```python
from build123d import *

# Parameters (mm, degrees)
SKETCH1_W           = 86.35
SKETCH1_H           = 86
SKETCH1_R           = 2.05
BOSS_EXTRUDE1_DEPTH = 3.175
FILLET1_R           = 4
SKETCH2_R           = 7.05
SKETCH2_R_2         = 12
CUT_EXTRUDE1_DEPTH  = 3.18


with BuildPart() as part:
    # Sketch1 → Boss-Extrude1 (new body)
    with BuildSketch(Plane(origin=(0, 0, 0), x_dir=(1, 0, 0), z_dir=(0, 1, 0))):
        Rectangle(SKETCH1_W, SKETCH1_H)
        with Locations(Location((37.675, 35, 0), (0, 0, 270))):
            Circle(SKETCH1_R, mode=Mode.SUBTRACT)
        with Locations(Location((37.675, 26.832661921, 0), (0, 0, 270))):
            Circle(SKETCH1_R, mode=Mode.SUBTRACT)
        with Locations(Location((37.675, 18.665323842, 0), (0, 0, 270))):
            Circle(SKETCH1_R, mode=Mode.SUBTRACT)
        with Locations(Location((37.675, 10.497985763, 0), (0, 0, 270))):
            Circle(SKETCH1_R, mode=Mode.SUBTRACT)
        with Locations(Location((37.675, 2.330647684, 0), (0, 0, 270))):
            Circle(SKETCH1_R, mode=Mode.SUBTRACT)
        with Locations(Location((37.675, -5.836690395, 0), (0, 0, 270))):
            Circle(SKETCH1_R, mode=Mode.SUBTRACT)
        with Locations(Location((37.675, -14.004028475, 0), (0, 0, 270))):
            Circle(SKETCH1_R, mode=Mode.SUBTRACT)
        with Locations(Location((37.675, -22.171366554, 0), (0, 0, 270))):
            Circle(SKETCH1_R, mode=Mode.SUBTRACT)
        with Locations(Location((37.675, -30.338704633, 0), (0, 0, 270))):
            Circle(SKETCH1_R, mode=Mode.SUBTRACT)
        with Locations(Location((37.675, -38.506042712, 0), (0, 0, 270))):
            Circle(SKETCH1_R, mode=Mode.SUBTRACT)
        with Locations(Location((-37.675, -38.506042712, 0), (0, 0, 90))):
            Circle(SKETCH1_R, mode=Mode.SUBTRACT)
        with Locations(Location((-37.675, -30.338704633, 0), (0, 0, 90))):
            Circle(SKETCH1_R, mode=Mode.SUBTRACT)
        with Locations(Location((-37.675, -22.171366554, 0), (0, 0, 90))):
            Circle(SKETCH1_R, mode=Mode.SUBTRACT)
        with Locations(Location((-37.675, -14.004028475, 0), (0, 0, 90))):
            Circle(SKETCH1_R, mode=Mode.SUBTRACT)
        with Locations(Location((-37.675, -5.836690395, 0), (0, 0, 90))):
            Circle(SKETCH1_R, mode=Mode.SUBTRACT)
        with Locations(Location((-37.675, 2.330647684, 0), (0, 0, 90))):
            Circle(SKETCH1_R, mode=Mode.SUBTRACT)
        with Locations(Location((-37.675, 10.497985763, 0), (0, 0, 90))):
            Circle(SKETCH1_R, mode=Mode.SUBTRACT)
        with Locations(Location((-37.675, 18.665323842, 0), (0, 0, 90))):
            Circle(SKETCH1_R, mode=Mode.SUBTRACT)
        with Locations(Location((-37.675, 26.832661921, 0), (0, 0, 90))):
            Circle(SKETCH1_R, mode=Mode.SUBTRACT)
        with Locations(Location((-37.675, 35, 0), (0, 0, 90))):
            Circle(SKETCH1_R, mode=Mode.SUBTRACT)
    extrude(amount=BOSS_EXTRUDE1_DEPTH)

    # Fillet1
    fillet1_edges = [part.edges().sort_by_distance(p)[0] for p in [
        (43.175, 1.5875, 43),
        (-43.175, 1.5875, 43),
        (-43.175, 1.5875, -43),
        (43.175, 1.5875, -43),
    ]]
    fillet(fillet1_edges, radius=FILLET1_R)

    # Sketch2 → Cut-Extrude1 (cut)
    with BuildSketch(Plane(origin=(0, 3.175, 0), x_dir=(1, 0, 0), z_dir=(0, 1, 0))):
        with Locations(Location((-17.9, 23, 0), (0, 0, 270))):
            Circle(SKETCH2_R)
        with Locations(Location((17.9, 23, 0), (0, 0, 270))):
            Circle(SKETCH2_R)
        with Locations(Location((0, -20.993410297, 0), (0, 0, 270))):
            Circle(SKETCH2_R_2)
        with BuildLine():
            Line((-17.9, -7.043410297), (-14.9, -7.043410297))
            ThreePointArc((-14.9, -7.043410297), (-12.85, -4.993410297), (-14.9, -2.943410297))
            Line((-14.9, -2.943410297), (-17.9, -2.943410297))
            ThreePointArc((-17.9, -2.943410297), (-19.95, -4.993410297), (-17.9, -7.043410297))
        make_face()
        with BuildLine():
            Line((17.1, -2.943410297), (14.1, -2.943410297))
            ThreePointArc((14.1, -2.943410297), (12.05, -4.993410297), (14.1, -7.043410297))
            Line((14.1, -7.043410297), (17.1, -7.043410297))
            ThreePointArc((17.1, -7.043410297), (19.15, -4.993410297), (17.1, -2.943410297))
        make_face()
        with BuildLine():
            Line((14.1, -34.943410297), (17.1, -34.943410297))
            ThreePointArc((17.1, -34.943410297), (19.15, -36.993410297), (17.1, -39.043410297))
            Line((17.1, -39.043410297), (14.1, -39.043410297))
            ThreePointArc((14.1, -39.043410297), (12.05, -36.993410297), (14.1, -34.943410297))
        make_face()
        with BuildLine():
            Line((-17.9, -34.943410297), (-14.9, -34.943410297))
            ThreePointArc((-14.9, -34.943410297), (-12.85, -36.993410297), (-14.9, -39.043410297))
            Line((-14.9, -39.043410297), (-17.9, -39.043410297))
            ThreePointArc((-17.9, -39.043410297), (-19.95, -36.993410297), (-17.9, -34.943410297))
        make_face()
    extrude(amount=-CUT_EXTRUDE1_DEPTH, mode=Mode.SUBTRACT)


solid = part.part
```
Source: CAD feature listing. Evaluate the final solid. Frame: model axes, mm. A direction names the side the tool comes from. Give positions to 0.01 mm unless a question says otherwise; leave off trailing zeros. Write each loop counter-clockwise with the first axis right and the second up, starting at its lowest first coordinate (ties: lowest second). Pieces come first, ordered by that corner, then holes.
1. Section query D-D (z = -1.5). Return the cut outline in (x, y) (3 decimals), then the cut area to 3 significant figures.
2. Section query B-B (z = -35). Return the cut outline in (x, y) (3 decimals), then the cut area to 3 significant figures.
3. Material intervals for line 1 along X through (y, z) = (1.2, -35) (3 decimals); line 2 along Z through (x, y) = (0.5, 1.2); line 3 along X through (y, z) = (3, 13.5) (3 decimals), sorted ascending.
4. Pull-direction query (X, two-part tool) for faces 1 (the face through (-1, 2, -43)), 2 (the face through (-43.175, 2, 1)), 3 (the face through (35.856, 1.565, 23.117)); classes: +X half, -X half, draft (parallel to the pull), parting line (faces both ways), or undercut.
5. Section query A-A (x = 0). Return the cut outline in (y, z) (3 decimals), then the cut area to 3 significant figures.
6. Section query C-C (z = 26). Return the cut outline in (x, y) (3 decimals), then the cut area to 3 significant figures.
7. Access query for faces 4 (the face through (-12.85, 1.61, 36.95)), 5 (the face through (41.97, 1.61, 41.86)). Directions: +Z, -Z, +X, -X, +Y, -Y. A direction counts if a zero-diameter tool reaches every point of the face in a straight line with its end or side. Return the directions, or none.
Output values:
1. outline: (-43.175, 0) - (-39.549, 0) - (-39.549, 3.175) - (-43.175, 3.175) - close; (-35.801, 0) - (35.801, 0) - (35.801, 3.175) - (-35.801, 3.175) - close; (39.549, 0) - (43.175, 0) - (43.175, 3.175) - (39.549, 3.175) - close
1. area: 250 mm2
2. outline: (-43.175, 0) - (-39.725, 0) - (-39.725, 3.175) - (-43.175, 3.175) - close; (-35.625, 0) - (35.625, 0) - (35.625, 3.175) - (-35.625, 3.175) - close; (39.725, 0) - (43.175, 0) - (43.175, 3.175) - (39.725, 3.175) - close
2. area: 248 mm2
3. line 1: x = -43.175 to -39.725, -35.625 to 35.625, 39.725 to 43.175
3. line 2: z = -43 to 9, 32.98 to 43
3. line 3: x = -43.175 to -39.662, -35.688 to -9.373, 9.373 to 35.688, 39.662 to 43.175
4. face 1: draft
4. face 2: -X half
4. face 3: undercut
5. outline: (0, -43) - (3.175, -43) - (3.175, 8.993) - (0, 8.993) - close; (0, 32.993) - (3.175, 32.993) - (3.175, 43) - (0, 43) - close
5. area: 197 mm2
6. outline: (-43.175, 0) - (-10.906, 0) - (-10.906, 3.175) - (-43.175, 3.175) - close; (10.906, 0) - (43.175, 0) - (43.175, 3.175) - (10.906, 3.175) - close
6. area: 205 mm2
7. face 4: +Y, -Y
7. face 5: +Z, +X, +Y, -Y
